Source: CAD feature listing. Evaluate the final solid. Frame: model axes, mm. Face numbers are marked on the shaded views. A direction names the side the tool comes from. Give positions to 0.01 mm unless a question says otherwise; leave off trailing zeros. Order: outer loops, then holes, each group sorted by start corner. A loop starts at its lowest first (then second) coordinate and runs counter-clockwise, first axis right, second up. Notation, with made-up numbers: M 67.25,-30 L 81.25,-30 A8 ccw 81.25,-20 Z; hole C 62.5,-17 d7. An arc over 180 degrees is marked long. Use CSV: the item, a comma, the result in double quotes. Start each with the question number.
Item 1: Section query D-D on z = 20.5. Return loops of the section in (x, y).
Item 2: Section query B-B on z = -6. Return loops of the section in (x, y).
Item 3: Section query A-A on y = 35. Return loops of the section in (x, z), and give its area (3 significant figures).
Item 4: Section query C-C on x = 0. Return loops of the section in (y, z), and give its area (3 significant figures).
Item 5: Ray query, probe 1 along Y at (x, z) = (0, 7); probe 2 along Z at (x, y) = (-20, -105); probe 3 along Z at (x, y) = (-15, 5). Return the intervals inside material, ascending. Write a range as from..to.
Item 6: Pull-direction query (X, two-part tool) for the marked faces 4, 5 and 6; classes: +X half, -X half, draft (parallel to the pull), parting line (faces both ways), or undercut.
Item 7: Access query for the marked faces 1, 2 and 3. Directions: +Z, -Z, +X, -X, +Y, -Y. A direction counts if a zero-diameter tool reaches every point of the face in a straight line with its end or side. Return the directions, or none.
Item 8: First-contact query: pin 1 (3 mm diameter, centred on x = -14, y = -77, fed in from -Z); pin 2 (9 mm diameter, centred on x = 7, y = -106, fed in from -Z). Flat tips, straight axial feed; report the tip coordinate or a pass-through.
from build123d import *

# Parameters (mm, degrees)
F0_W     = 50
F0_H     = 230
F1_DEPTH = 27
F2_W     = 30
F2_H     = 10
F2_H_2   = 16
F3_DEPTH = 50
F5_D     = 21


with BuildPart() as f1:
    # F0 (on Top) → F1 (new body)
    with BuildSketch(Plane.XY):
        Rectangle(F0_W, F0_H)
    extrude(amount=F1_DEPTH)

    # F2 (on face) → F3 (join, through all)
    with BuildSketch(Plane(origin=(-25, 0, 0), x_dir=(0, -1, 0), z_dir=(-1, 0, 0))):
        with Locations((100, -5)):
            Rectangle(F2_W, F2_H)
        with Locations((-100, -8)):
            Rectangle(F2_W, F2_H_2)
    extrude(amount=-F3_DEPTH)

    # F5 (through all)
    with Locations(Plane.XY.offset(27)):
        with Locations((0, 35)):
            Hole(F5_D / 2)


solid = f1.part
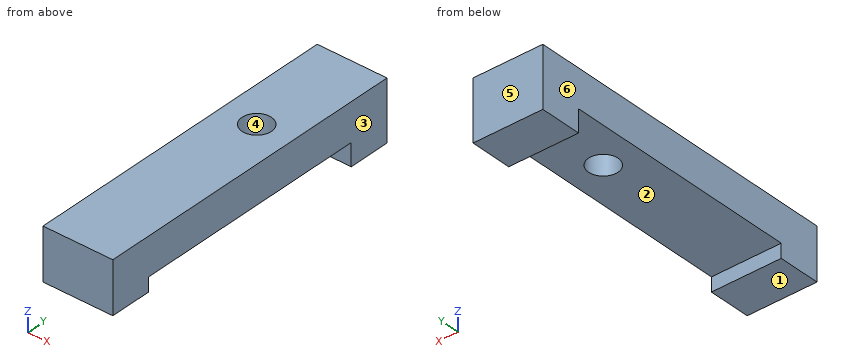
Verdict:
1,outline,"M -25,-115 L 25,-115 L 25,115 L -25,115 Z; hole C 0,35 d21"
2,outline,"M -25,-115 L 25,-115 L 25,-85 L -25,-85 Z; M -25,85 L 25,85 L 25,115 L -25,115 Z"
3,outline,"M -25,0 L -10.5,0 L -10.5,27 L -25,27 Z; M 10.5,0 L 25,0 L 25,27 L 10.5,27 Z"
3,area,"783 mm2"
4,outline,"M -115,-10 L -85,-10 L -85,0 L 24.5,0 L 24.5,27 L -115,27 Z; M 45.5,0 L 85,0 L 85,-16 L 115,-16 L 115,27 L 45.5,27 Z"
4,area,"6,420 mm2"
5,probe 1,"-115..24.5, 45.5..115"
5,probe 2,"-10..27"
5,probe 3,"0..27"
6,face 4,"undercut"
6,face 5,"draft"
6,face 6,"-X half"
7,face 1,"-Z, +X, -X, -Y"
7,face 2,"-Z, +X, -X"
7,face 3,"+Z, -Z, +X, +Y, -Y"
8,pin 1,"z = 0"
8,pin 2,"z = -10"
